```python
from build123d import *

# Parameters (mm, degrees)
SKETCH1_R           = 11.291730028
SKETCH1_R_2         = 8
BOSS_EXTRUDE1_DEPTH = 10
SKETCH2_W           = 22.583460056
SKETCH2_H           = 31.840111269
BOSS_EXTRUDE2_DEPTH = 20
CUT_EXTRUDE1_REACH  = 40.075
SKETCH3_R           = 8


with BuildPart() as part:
    # Sketch1 → Boss-Extrude1 (new body)
    with BuildSketch(Plane.XY):
        Circle(SKETCH1_R)
        Circle(SKETCH1_R_2, mode=Mode.SUBTRACT)
    extrude(amount=BOSS_EXTRUDE1_DEPTH)

    # Sketch2 → Boss-Extrude2 (add)
    with BuildSketch(Plane.XY.offset(10)):
        with Locations((0, -4.628325607)):
            Rectangle(SKETCH2_W, SKETCH2_H)
    extrude(amount=BOSS_EXTRUDE2_DEPTH)

    # Sketch3 → Cut-Extrude1 (cut, up to next)
    with BuildSketch(Plane.XY.offset(30), mode=Mode.PRIVATE) as cut_extrude1_sk1:
        Circle(SKETCH3_R)
    cut_extrude1_tool1 = extrude(cut_extrude1_sk1.sketch, amount=-CUT_EXTRUDE1_REACH, mode=Mode.PRIVATE) & part.part
    add(cut_extrude1_tool1.solids().sort_by_distance((0, 0, 30))[0], mode=Mode.SUBTRACT)


solid = part.part
```
Can you work these out from the model? Positions are in its coordinate system, mm. A direction names the side the tool comes from. Round coordinates to 2 decimals unless told otherwise and drop trailing zeros. Loops run counter-clockwise (first coordinate to the right, second up) from the corner with the lowest first, then second, coordinate; pieces in that order, holes last.
Item 1: Please list where these lines run through material, in increasing order: L1, parallel to Y at x = 0, z = 15.5; L2, parallel to X at y = -7, z = 15.25; L3, parallel to Y at x = 7, z = 20.25.
Item 2: Suppose I cut it at B-B, the plane x = 1.25. Write out the boundary of the cut face in (y, z).
Item 3: Suppose I cut it at A-A, the plane y = -3. Write out the boundary of the cut face in (x, z).
Item 4: Which directions (+Z, -Z, +X, -X, +Y, -Y) give clear straight access to the entire face, cutting with the end or side of a thin tool? Please do faces 1 (the cylindrical face through (-8.96, -6.87, 4.93)), 2 (the flat face through (9, 9, 10)), 3 (the flat face through (-9, 9, 10)).
Item 5: Will this pin go through, and if not, where does the flat tip stop? pin 1 Ø8 at (x, z) = (0.5, 3.5) entering from -Y.
Item 6: Suppose I cut it at C-C, the plane z = 27.75. Write out the boundary of the cut face in (x, y), then the cut area to 3 significant figures.
Item 7: Suppose I cut it at D-D, the plane z = 7. Write out the boundary of the cut face in (x, y).
Item 8: If we mould it in two halves opening along X, with no side actions, what happens to faces 4 (the flat face through (11.292, -5, 20)), 5 (the cylindrical face through (-1.73, -7.81, 15.21)), 6 (the flat face through (-3, -8, 30))? For each: +X half, -X half, draft (parallel to the pull), parting line (faces both ways), or undercut.
Reported:
1. L1: y = -20.55 to -8, 8 to 11.29
1. L2: x = -11.29 to -3.87, 3.87 to 11.29
1. L3: y = -20.55 to -3.87, 3.87 to 11.29
2. outline: (-20.55, 10) - (-11.22, 10) - (-11.22, 0) - (-7.9, 0) - (-7.9, 30) - (-20.55, 30) - close; (7.9, 0) - (11.22, 0) - (11.22, 10) - (11.29, 10) - (11.29, 30) - (7.9, 30) - close
3. outline: (-11.29, 10) - (-10.89, 10) - (-10.89, 0) - (-7.42, 0) - (-7.42, 30) - (-11.29, 30) - close; (7.42, 0) - (10.89, 0) - (10.89, 10) - (11.29, 10) - (11.29, 30) - (7.42, 30) - close
4. face 1: -Z
4. face 2: -Z, +X, +Y
4. face 3: -Z, -X, +Y
5. pin 1: stops at y = -11.29
6. outline: (-11.29, -20.55) - (11.29, -20.55) - (11.29, 11.29) - (-11.29, 11.29) - close; hole circle Ø16 at (0, 0)
6. area: 518 mm2
7. outline: circle Ø22.58 at (0, 0); hole circle Ø16 at (0, 0)
8. face 4: +X half
8. face 5: undercut
8. face 6: draft
